from build123d import *

# Parameters (mm, degrees)
FILLET1_R = 2


with BuildPart() as part:
    # Sketch1 → Revolve1 (revolve)
    with BuildSketch(Plane(origin=(0, 0, 0), x_dir=(0, 0, -1), z_dir=(1, 0, 0))):
        Polygon((0, 10), (25, 10), (25, 21), (20, 21), (20, 18), (5, 18), (5, 21), (0, 21), align=None)
    revolve(axis=Axis((0, 0, 0), (0, 0, -1)))

    # Fillet1
    fillet1_edges = [part.edges().sort_by_distance(p)[0] for p in [
        (0, -21, 0),
        (0, -21, -5),
        (0, -21, -20),
        (0, -21, -25),
    ]]
    fillet(fillet1_edges, radius=FILLET1_R)


solid = part.part
Could you check a few things on this model? Use its own coordinates, in mm. A direction names the side the tool comes from. Give positions to 0.01 mm unless a question says otherwise; leave off trailing zeros. Order: outer loops, then holes, each group sorted by start corner. A loop starts at its lowest first (then second) coordinate and runs counter-clockwise, first axis right, second up. Notation, with made-up numbers: (-13, 0.5) - (40, 0.5) arc R29 cw to (40, 26.5) - close; hole circle Ø5 at (5.25, 78). An arc over 180 degrees is marked (long way). One line per question, with ' | ' between items. Start each with the question number.
Item 1: Thinking about a two-plate mould opening in Y: for faces 3 (the flat face through (-17, -7, -5)), 4 (the cylindrical face through (-9.76, -2.17, -12.68)), 5 (the cylindrical face through (6.31, 20.03, -2.49)), which applies, pulls with the +Y half, pulls with the -Y half, needs draft (parallel to the pull), parting line crosses it, or undercut?
Item 2: I want a section at D-D on z = -4.25. Write out the boundary of the cut face in (x, y).
Item 3: I want a section at A-A on x = 0. Write out the boundary of the cut face in (y, z), then the cut area to 3 significant figures.
Item 4: I want a section at C-C on z = -16.5. Write out the boundary of the cut face in (x, y).
Item 5: I need wall thicknesses on probe 1 along Z at (x, y) = (18, -4); probe 2 along X at (y, z) = (0, -15); probe 3 along X at (y, z) = (-3, -16). Which ranges of each line are inside material? Lowest first, please. Write a range as [from, to].
Item 6: For faces 1 (the flat face through (-8, 8, 0)), 2 (the flat face through (-17, 7, -20)), which set-ups out of +Z, -Z, +X, -X, +Y, -Y let a thin tool reach every point of the face, with its end or its side?
Item 7: I'm going to push flat-ended pins straight in: pin 1 Ø3 at (y, z) = (16, -9) entering from -X; pin 2 Ø8 at (x, z) = (5, -5.5) entering from +Y; pin 3 Ø12 at (x, z) = (8.5, -12.5) entering from +Y. Where does each tip first touch, or does it pass through?
Verdict:
1) face 3: needs draft | face 4: undercut | face 5: parting line crosses it
2) outline: circle Ø41.12 at (0, 0); hole circle Ø20 at (0, 0)
3) outline: (-21, -23) arc R2 ccw to (-19, -25) - (-10, -25) - (-10, 0) - (-19, 0) arc R2 ccw to (-21, -2) - (-21, -3) arc R2 ccw to (-19, -5) - (-18, -5) - (-18, -20) - (-19, -20) arc R2 ccw to (-21, -22) - close; (10, -25) - (19, -25) arc R2 ccw to (21, -23) - (21, -22) arc R2 ccw to (19, -20) - (18, -20) - (18, -5) - (19, -5) arc R2 ccw to (21, -3) - (21, -2) arc R2 ccw to (19, 0) - (10, 0) - close | area: 453 mm^2
4) outline: circle Ø36 at (0, 0); hole circle Ø20 at (0, 0)
5) probe 1: [-25, -20], [-5, 0] | probe 2: [-18, -10], [10, 18] | probe 3: [-17.75, -9.54], [9.54, 17.75]
6) face 1: +Z, +X, -X, +Y, -Y | face 2: none
7) pin 1: x = -10.67 | pin 2: y = 20.92 | pin 3: y = 17.83
